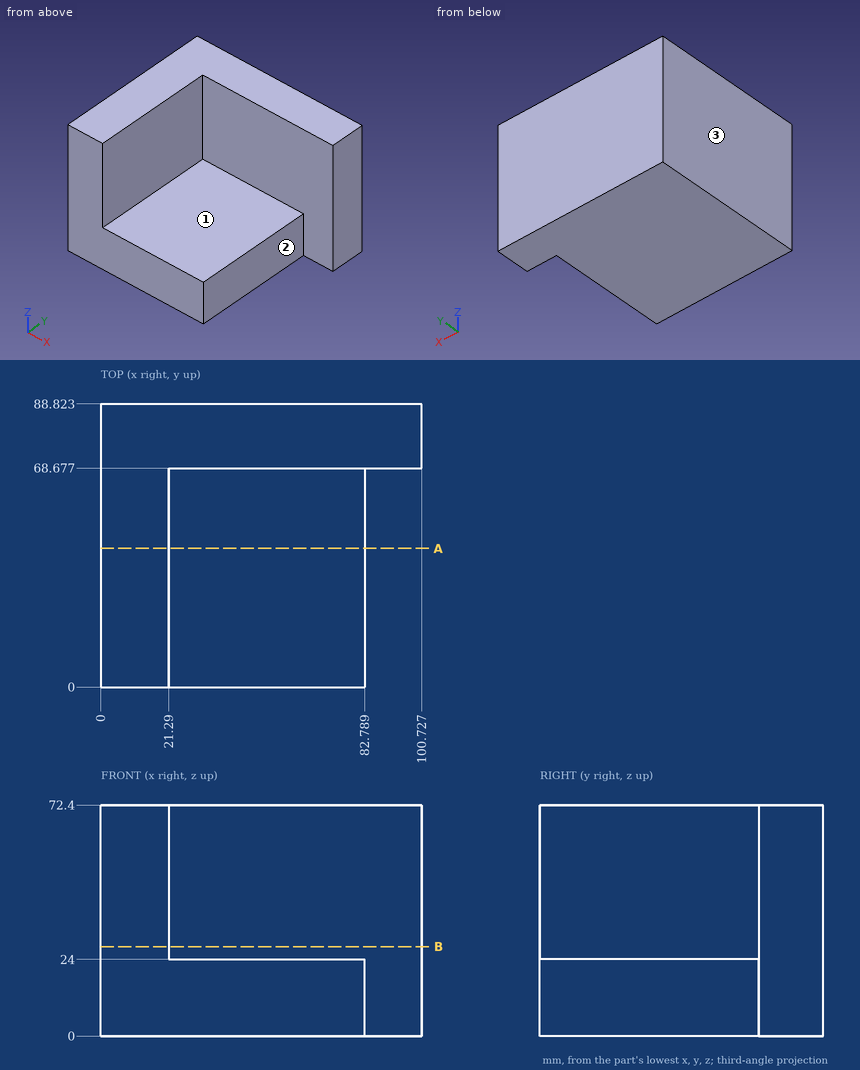
Could you check a few things on this drawing? It's one solid part, dimensions in mm from its lowest x, y, z. A direction names the side the tool comes from. Coordinates: 2 decimals unless noted, no trailing zeros. Order: outer loops, then holes, each group sorted by start corner. A loop starts at its lowest first (then second) coordinate and runs counter-clockwise, first axis right, second up.
1) Imagine slicing it at B-B on z = 28. List the corners of the cut face in (x, y) for me, and give its area (3 significant figures).
2) I need wall thicknesses on line 1 (Z direction, x = 24, y = 25); line 2 (X direction, y = 53, z = 30.5); line 3 (Y direction, x = 74, z = 29). Which ranges of each line are inside material? Lowest first, please.
3) Which directions (+Z, -Z, +X, -X, +Y, -Y) give clear straight access to the entire face, cutting with the end or side of a thin tool? Please do the marked faces 1, 2 and 3.
4) Imagine slicing it at A-A on y = 43.5. List the corners of the cut face in (x, z) for me.
5) Will these pins go through, and if not, where does the flat tip stop? pin 1 (1.5 mm diameter, centred on x = 46, z = 56.5, fed in from -Y); pin 2 (24 mm diameter, centred on y = 26, z = 53.5, fed in from +X); pin 3 (8 mm diameter, centred on x = 29, y = 21.5, fed in from -Z); pin 4 (12 mm diameter, centred on y = 17.5, z = 10.5, fed in from +X).
Response values:
1. outline: (0, 0) - (21.29, 0) - (21.29, 68.68) - (100.73, 68.68) - (100.73, 88.82) - (0, 88.82) - close
1. area: 3,490 mm2
2. line 1: z = 0 to 24
2. line 2: x = 0 to 21.29
2. line 3: y = 68.68 to 88.82
3. face 1: +Z, +X, -Y
3. face 2: +Z, -Z, +X, -Y
3. face 3: +Z, -Z, -X, +Y, -Y
4. outline: (0, 0) - (82.79, 0) - (82.79, 24) - (21.29, 24) - (21.29, 72.4) - (0, 72.4) - close
5. pin 1: stops at y = 68.68
5. pin 2: stops at x = 21.29
5. pin 3: stops at z = 0
5. pin 4: stops at x = 82.79
